The listing builds one solid part. Answer for the finished solid, in the listing's coordinates (mm). A direction names the side the tool comes from. Coordinates: 2 decimals unless noted, no trailing zeros. Loops run counter-clockwise (first coordinate to the right, second up) from the corner with the lowest first, then second, coordinate; pieces in that order, holes last. Notation, with made-up numbers: (67, 15) - (87, 15) arc R23 cw to (87, 35) - close; hole circle Ø9 at (40, -31). An arc over 180 degrees is marked (long way). Return JSON: item names as keys, results as strings. Group by question number.
1. Which of the six approach directions +Z, -Z, +X, -X, +Y, -Y give full straight-line access (tool end or side, diameter ignored) to faces 4 (the face through (54.974, -31.783, 2.962)), 5 (the face through (-40, 22, 5.842))?
2. Section C-C (y = 48.5) is taken. Write down the section's boundary in (x, z), and give its area (3 significant figures).
3. Section A-A (x = 0) is taken. Write down the section's boundary in (y, z) (3 decimals).
4. Section D-D (z = 2) is taken. State how many separate pieces and enclosed holes the cut face has, and give its area (3 significant figures).
5. Section B-B (y = 0) is taken. Write down the section's boundary in (x, z), and give its area (3 significant figures).
6. The mould has two halves that part along X. Classify faces 1 (the face through (50.96, 25.76, 2.88)), 2 (the face through (-60.934, 34.148, 2.88)), 3 (the face through (0, 69.85, 3)): pulls with the +X half, pulls with the -X half, needs draft (parallel to the pull), parting line crosses it, or undercut.
7. Each of these flat-tipped pins is pushed along its axis until it touches: P1, Ø3, axis at y = 46.5, z = 4, coming from the -X side; P2, Ø2, axis at y = 41.5, z = 1.5, coming from the +X side; P3, Ø1.5, axis at y = 18, z = 5, coming from the -X side. Where does it stop, or does it pass through?
8. Find the intervals of material crossed by line 1 along Y through (x, z) = (0, 3.6) (3 decimals); line 2 along X through (y, z) = (-58, 3.15); line 3 along X through (y, z) = (-50, 0.3), in increasing order.
```python
from build123d import *

# Parameters (mm, degrees)
SKETCH1_R           = 44.45
SKETCH1_R_2         = 3.175
BOSS_EXTRUDE1_DEPTH = 5.842
FILLET5_R           = 25.4
SKETCH3_R           = 69.85
SKETCH3_R_2         = 63.5
BOSS_EXTRUDE3_DEPTH = 5.842
FILLET7_R           = 1.5875
SKETCH5_W           = 18.542
SKETCH5_H           = 25.4
BOSS_EXTRUDE4_DEPTH = 5.842
CIRPATTERN1_COUNT   = 3
FILLET8_R           = 1.5875
CUT_EXTRUDE7_DEPTH  = 99.955414168
CIRPATTERN2_COUNT   = 3
FILLET9_R           = 3.175


with BuildPart() as part:
    # Sketch1 → Boss-Extrude1 (new body)
    with BuildSketch(Plane.XY):
        with BuildLine():
            ThreePointArc((-53.551878894, 19.957924914), (-49.493351826, -28.575), (-9.491869465, -56.35625))
            ThreePointArc((-9.491869465, -56.35625), (0, -66.675), (9.491869465, -56.35625))
            ThreePointArc((9.491869465, -56.35625), (49.493351826, -28.575), (53.551878894, 19.957924914))
            ThreePointArc((53.551878894, 19.957924914), (57.742243797, 33.3375), (44.06000943, 36.398325086))
            ThreePointArc((44.06000943, 36.398325086), (0, 57.15), (-44.06000943, 36.398325086))
            ThreePointArc((-44.06000943, 36.398325086), (-57.742243797, 33.3375), (-53.551878894, 19.957924914))
        make_face()
        Circle(SKETCH1_R, mode=Mode.SUBTRACT)
        with Locations((49.493351826, 28.575)):
            Circle(SKETCH1_R_2, mode=Mode.SUBTRACT)
        with Locations((0, -57.15)):
            Circle(SKETCH1_R_2, mode=Mode.SUBTRACT)
        with Locations((-49.493351826, 28.575)):
            Circle(SKETCH1_R_2, mode=Mode.SUBTRACT)
    extrude(amount=BOSS_EXTRUDE1_DEPTH)

    # Fillet5
    fillet5_edges = [part.edges().sort_by_distance(p)[0] for p in [
        (44.06000943, 36.398325086, 2.921),
        (53.551878894, 19.957924914, 2.921),
        (9.491869465, -56.35625, 2.921),
        (-9.491869465, -56.35625, 2.921),
        (-53.551878894, 19.957924914, 2.921),
        (-44.06000943, 36.398325086, 2.921),
    ]]
    fillet(fillet5_edges, radius=FILLET5_R)

    # Sketch3 → Boss-Extrude3 (add)
    with BuildSketch(Plane(origin=(0, 0, 0), x_dir=(-1, 0, 0), z_dir=(0, 0, -1))):
        Circle(SKETCH3_R)
        Circle(SKETCH3_R_2, mode=Mode.SUBTRACT)
    extrude(amount=-BOSS_EXTRUDE3_DEPTH)

    # Fillet7
    fillet7_edges = [part.edges().sort_by_distance(p)[0] for p in [
        (58.345991594, 25.059833697, 2.921),
        (50.875448393, 37.999194081, 2.921),
        (-7.470543201, -63.059027778, 2.921),
        (7.470543201, -63.059027778, 2.921),
        (-50.875448393, 37.999194081, 2.921),
        (-58.345991594, 25.059833697, 2.921),
    ]]
    fillet(fillet7_edges, radius=FILLET7_R)

    # Sketch5 → Boss-Extrude4 (add)
    with BuildSketch(Plane.XY.offset(5.842)):
        with Locations((0, 57.15)):
            Rectangle(SKETCH5_W, SKETCH5_H)
    boss_extrude4 = extrude(amount=-BOSS_EXTRUDE4_DEPTH)

    # CirPattern1: Boss-Extrude4 ×3 about axis
    cirpattern1_axis = Axis((0, 0, 0), (0, 0, 1))
    for i in range(1, CIRPATTERN1_COUNT):
        add(boss_extrude4.rotate(cirpattern1_axis, i * 360 / CIRPATTERN1_COUNT))

    # Fillet8
    # the kernel refuses this fillet: 1.5875 mm, written as the material it takes off along each edge
    with BuildSketch(Plane(origin=(65.127374454, -26.896078482, 8.984658812), x_dir=(-0.8660254037844379, 0.500000000000001, 0), z_dir=(0, 0, -1)), Plane(origin=(-9.271, 69.85, 8.984658812), x_dir=(0, -1, 0), z_dir=(0, 0, -1))) as fillet8_piece_1:
        with BuildLine():
            CenterArc((1.5875, -1.257063525), FILLET8_R, 127.641167987, 52.358832013)
            Line((0, -1.257063525), (-0.03175, -1.257063525))
            Line((-0.03175, -1.257063525), (-0.03175, 0))
            Line((-0.03175, 0), (0, 0.03175))
            ThreePointArc((0, 0.03175), (0.30899554, 0.03175), (0.598600902, 0.02514127))
            Line((0.598600902, 0.02514127), (0.617991081, 0))
        make_face()
    extrude(amount=12.127317624, mode=Mode.SUBTRACT)
    with BuildSketch(Plane(origin=(55.856374454, -42.953921518, 8.984658812), x_dir=(0.5000000000000007, 0.8660254037844382, 0), z_dir=(0, 0, -1)), Plane(origin=(-65.127374454, -26.896078482, 8.984658812), x_dir=(0.5000000000000024, -0.8660254037844373, 0), z_dir=(0, 0, -1)), Plane(origin=(9.271, 69.85, 8.984658812), x_dir=(-1, 0, 0), z_dir=(0, 0, -1))) as fillet8_piece_2:
        with BuildLine():
            CenterArc((1.257063525, -1.5875), FILLET8_R, 90, 52.358832013)
            Line((0, -0.617991081), (-0.02514127, -0.598600902))
            ThreePointArc((-0.02514127, -0.598600902), (-0.03175, -0.30899554), (-0.03175, 0))
            Line((-0.03175, 0), (0, 0.03175))
            Line((0, 0.03175), (1.257063525, 0.03175))
            Line((1.257063525, 0.03175), (1.257063525, 0))
        make_face()
    extrude(amount=12.127317624, mode=Mode.SUBTRACT)
    with BuildSketch(Plane(origin=(-55.856374454, -42.953921518, 8.984658812), x_dir=(-0.5, 0.8660254037844386, 0), z_dir=(0, 0, -1))) as fillet8_piece_3:
        with BuildLine():
            CenterArc((1.257063525, 1.5875), FILLET8_R, 217.641167987, 52.358832013)
            Line((0, 0.617991081), (-0.02514127, 0.598600902))
            ThreePointArc((-0.02514127, 0.598600902), (-0.03175, 0.30899554), (-0.03175, 0))
            Line((-0.03175, 0), (0, -0.03175))
            Line((0, -0.03175), (1.257063525, -0.03175))
            Line((1.257063525, -0.03175), (1.257063525, 0))
        make_face()
    extrude(amount=12.127317624, mode=Mode.SUBTRACT)

    # Sketch7 → Cut-Extrude7 (cut, through all)
    with BuildSketch(Plane.XY.offset(5.842)):
        with BuildLine():
            Line((2.7225625, 63.5), (-2.7225625, 63.5))
            ThreePointArc((-2.7225625, 63.5), (-3.061316502, 63.640316502), (-2.921, 63.3015625))
            Line((-2.921, 63.3015625), (-2.921, 50.9984375))
            ThreePointArc((-2.921, 50.9984375), (-3.061316502, 50.659683498), (-2.7225625, 50.8))
            Line((-2.7225625, 50.8), (2.7225625, 50.8))
            ThreePointArc((2.7225625, 50.8), (3.061316502, 50.659683498), (2.921, 50.9984375))
            Line((2.921, 50.9984375), (2.921, 63.3015625))
            ThreePointArc((2.921, 63.3015625), (3.061316502, 63.640316502), (2.7225625, 63.5))
        make_face()
    cut_extrude7 = extrude(amount=-CUT_EXTRUDE7_DEPTH, mode=Mode.SUBTRACT)

    # CirPattern2: Cut-Extrude7 ×3 about axis
    cirpattern2_axis = Axis((0, 0, 0), (0, 0, 1))
    for i in range(1, CIRPATTERN2_COUNT):
        add(cut_extrude7.rotate(cirpattern2_axis, i * 360 / CIRPATTERN2_COUNT), mode=Mode.SUBTRACT)

    # Fillet9
    # the kernel refuses this fillet: 3.175 mm, written as the material it adds along each edge
    with BuildSketch(Plane(origin=(9.271, 56.393005408, 5.842), x_dir=(0.9828671529049069, -0.18431538118291227, 0), z_dir=(0, 0, -1)), Plane(origin=(44.202275279, -36.225424223, 5.842), x_dir=(-0.6510553788650718, -0.7590302323694741, 0), z_dir=(0, 0, -1)), Plane(origin=(-53.473275279, -20.167581186, 5.842), x_dir=(-0.33181177403983686, 0.9433456135523905, 0), z_dir=(0, 0, -1))) as fillet9_piece_1:
        with BuildLine():
            CenterArc((2.635092544, -3.174201143), FILLET9_R, 91.285314708, 78.093465038)
            Line((-0.485510666, -2.588999807), (0, 0))
            ThreePointArc((0, 0), (1.281936913, -0.014379431), (2.563873827, 0))
        make_face()
    extrude(amount=5.842)
    with BuildSketch(Plane(origin=(9.271, 62.819571465, 5.842), x_dir=(0, -1, 0), z_dir=(0, 0, -1)), Plane(origin=(49.767844743, -39.438707251, 5.842), x_dir=(-0.8660254037844377, 0.5000000000000018, 0), z_dir=(0, 0, -1)), Plane(origin=(-59.038844743, -23.380864214, 5.842), x_dir=(0.8660254037844375, 0.500000000000002, 0), z_dir=(0, 0, -1))) as fillet9_piece_2:
        with BuildLine():
            CenterArc((3.792436103, -3.175), FILLET9_R, 90, 101.906534962)
            ThreePointArc((0.685744768, -3.830052632), (0.313529726, -1.920279918), (0, 0))
            Line((0, 0), (3.792436103, 0))
        make_face()
    extrude(amount=5.842)
    with BuildSketch(Plane(origin=(-9.271, 56.393005408, 5.842), x_dir=(-0.9828671529049081, -0.18431538118290586, 0), z_dir=(0, 0, -1))) as fillet9_piece_3:
        with BuildLine():
            CenterArc((2.635092544, 3.174201143), FILLET9_R, 190.621220255, 78.093465038)
            Line((-0.485510666, 2.588999807), (0, 0))
            ThreePointArc((0, 0), (1.281936913, 0.014379431), (2.563873827, 0))
        make_face()
    extrude(amount=5.842)
    with BuildSketch(Plane(origin=(-9.271, 62.819571465, 5.842), x_dir=(-0.9843471139890508, -0.17624062863433815, 0), z_dir=(0, 0, -1)), Plane(origin=(59.038844743, -23.380864214, 5.842), x_dir=(0.339544695418249, 0.9405899211735838, 0), z_dir=(0, 0, -1)), Plane(origin=(-49.767844743, -39.438707251, 5.842), x_dir=(0.6448024185707977, -0.7643492925392487, 0), z_dir=(0, 0, -1))) as fillet9_piece_4:
        with BuildLine():
            CenterArc((3.79368341, -3.173509537), FILLET9_R, 88.244328147, 101.906534962)
            Line((0.668381323, -3.733073533), (0, 0))
            ThreePointArc((0, 0), (1.945478672, 0.029809259), (3.890957343, 0))
        make_face()
    extrude(amount=5.842)
    with BuildSketch(Plane(origin=(53.473275279, -20.167581186, 5.842), x_dir=(0.8660254037844376, -0.5000000000000019, 0), z_dir=(0, 0, -1)), Plane(origin=(-44.202275279, -36.225424223, 5.842), x_dir=(-0.866025403784439, -0.49999999999999933, 0), z_dir=(0, 0, -1))) as fillet9_piece_5:
        with BuildLine():
            CenterArc((2.634129953, -3.175), FILLET9_R, 90, 78.093465038)
            ThreePointArc((-0.472561382, -2.519947368), (-0.22214762, -1.262624035), (0, 0))
            Line((0, 0), (2.634129953, 0))
        make_face()
    extrude(amount=5.842)


solid = part.part
```
The answers:
{
 "1": {"face 4": "+Z, -Z", "face 5": "+Z, +X, -X, +Y, -Y"},
 "2": {"outline": "(-50.27, 0) - (-40.99, 0) - (-40.99, 5.84) - (-50.27, 5.84) - close; (-30.23, 0) - (30.23, 0) - (30.23, 5.84) - (-30.23, 5.84) - close; (40.99, 0) - (50.27, 0) - (50.27, 5.84) - (40.99, 5.84) - close", "area": "462 mm2"},
 "3": {"outline": "(-69.85, 0) - (-60.325, 0) - (-60.325, 5.842) - (-69.85, 5.842) - close; (-53.975, 0) - (-44.45, 0) - (-44.45, 5.842) - (-53.975, 5.842) - close; (44.45, 0) - (50.8, 0) - (50.8, 5.842) - (44.45, 5.842) - close; (63.5, 0) - (69.85, 0) - (69.85, 5.842) - (63.5, 5.842) - close"},
 "4": {"separate pieces": "1", "enclosed holes": "13", "area": "7,240 mm2"},
 "5": {"outline": "(-69.85, 0) - (-63.5, 0) - (-63.5, 5.84) - (-69.85, 5.84) - close; (-57.15, 0) - (-44.45, 0) - (-44.45, 5.84) - (-57.15, 5.84) - close; (44.45, 0) - (57.15, 0) - (57.15, 5.84) - (44.45, 5.84) - close; (63.5, 0) - (69.85, 0) - (69.85, 5.84) - (63.5, 5.84) - close", "area": "223 mm2"},
 "6": {"face 1": "undercut", "face 2": "pulls with the -X half", "face 3": "needs draft"},
 "7": {"P1": "stops at x = -53.42", "P2": "stops at x = 56.91", "P3": "stops at x = -67.69"},
 "8": {"line 1": "y = -69.85 to -60.325, -53.975 to -44.45, 44.45 to 50.8, 63.5 to 69.85", "line 2": "x = -38.92 to -25.85, -12.12 to -3.06, 3.06 to 12.12, 25.85 to 38.92", "line 3": "x = -48.78 to -39.14, -27.68 to 27.68, 39.14 to 48.78"}
}
